Geometry: final body of the model. Coordinates: model frame, mm. Face numbers are marked on the shaded views. A direction names the side the tool comes from. Give positions to 0.01 mm unless a question says otherwise; leave off trailing zeros. Write each loop counter-clockwise with the first axis right and the second up, starting at its lowest first coordinate (ties: lowest second). Pieces come first, ordered by that corner, then holes. Notation, with made-up numbers: (27, 36) -> (65, 36) arc R15 cw to (65, 54) -> close; hole circle Ø7 at (16, 20). An arc over 180 degrees is marked (long way). Answer as a JSON object with one key per item and string values. Group by question number.
(1) Section query D-D on z = 5.25. Output: boundary loops of the cut face in (x, y), plus the area to 3 significant figures.
(2) Section query C-C on y = -4. Output: boundary loops of the cut face in (x, z), plus the area to 3 significant figures.
(3) Draft query along X for the marked faces 4, 5 and 6. Return one class per face: +X half, -X half, draft (parallel to the pull), parting line (faces both ways), or undercut.
(4) Material intervals for probe 1 along X at (y, z) = (-3, 3); probe 2 along Y at (x, z) = (5, 0.5); probe 3 along Z at (x, y) = (33.5, 5), sorted ascending.
(5) Contact query for flat-ended pins moving along their axis: pin 1 Ø5 at (x, z) = (22.5, 4) entering from +Y; pin 2 Ø1.9 at (x, y) = (32.5, 13.5) entering from -Z; pin 3 Ø3.5 at (x, y) = (12.5, 13.5) entering from +Z; pin 4 Ø17 at (x, y) = (13, 11.5) entering from +Z. Output: stop coordinate, or through.
(6) Section query B-B on y = 13.5. Output: boundary loops of the cut face in (x, z), plus the area to 3 significant figures.
(7) Section query A-A on x = 22.5. Output: boundary loops of the cut face in (y, z).
(8) Set-up query: the marked faces 1, 2 and 3. Return all of +Z, -Z, +X, -X, +Y, -Y with unobstructed straight access to the full face (end or side cutting, diameter ignored); none if empty.
from build123d import *

# Parameters (mm, degrees)
SALIENTE_EXTRUIR1_DEPTH = 45
REDONDEO1_R             = 2.5
CROQUIS2_R              = 2
CORTAR_EXTRUIR1_DEPTH   = 50.295030175
CROQUIS3_R              = 1.55
CORTAR_EXTRUIR2_DEPTH   = 53.242224302
CROQUIS4_W              = 45
CROQUIS4_H              = 18
SALIENTE_EXTRUIR2_DEPTH = 10
REDONDEO3_R             = 5
CROQUIS5_W              = 16
CROQUIS5_H              = 10
CORTAR_EXTRUIR3_DEPTH   = 53.242224302
REDONDEO4_R             = 5


with BuildPart() as part:
    # Croquis1 → Saliente-Extruir1 (new body)
    with BuildSketch(Plane(origin=(0, 0, 0), x_dir=(0, 0, -1), z_dir=(1, 0, 0))):
        Polygon((-9, -1.5), (9, -1.5), (9, 1.5), (9, 19.5), (6, 19.5), (6, 1.5), (-9, 1.5), align=None)
    extrude(amount=SALIENTE_EXTRUIR1_DEPTH)

    # Redondeo1
    redondeo1_edges = [part.edges().sort_by_distance(p)[0] for p in [
        (22.5, 1.5, -6),
    ]]
    fillet(redondeo1_edges, radius=REDONDEO1_R)

    # Croquis2 → Cortar-Extruir1 (cut, through all)
    with BuildSketch(Plane(origin=(0, 1.5, 0), x_dir=(1, 0, 0), z_dir=(0, 1, 0))):
        with Locations(Location((22.5, -4, 0), (0, 0, 270))):
            Circle(CROQUIS2_R)
    extrude(amount=-CORTAR_EXTRUIR1_DEPTH, mode=Mode.SUBTRACT)

    # Croquis3 → Cortar-Extruir2 (cut, through all)
    with BuildSketch(Plane(origin=(0, 0, -9), x_dir=(-1, 0, 0), z_dir=(0, 0, -1))):
        with Locations(Location((-32.5, 13.5, 0), (0, 0, 90))):
            Circle(CROQUIS3_R)
        with Locations((-12.5, 13.5)):
            Circle(CROQUIS3_R)
    extrude(amount=-CORTAR_EXTRUIR2_DEPTH, mode=Mode.SUBTRACT)

    # Croquis4 → Saliente-Extruir2 (add)
    with BuildSketch(Plane.XZ.offset(1.5)):
        with Locations((22.5, 0)):
            Rectangle(CROQUIS4_W, CROQUIS4_H)
    extrude(amount=SALIENTE_EXTRUIR2_DEPTH)

    # Redondeo3
    redondeo3_edges = [part.edges().sort_by_distance(p)[0] for p in [
        (45, -5, 9),
        (0, -5, 9),
    ]]
    fillet(redondeo3_edges, radius=REDONDEO3_R)

    # Croquis5 → Cortar-Extruir3 (cut, through all)
    with BuildSketch(Plane.XY.offset(9)):
        with Locations((22.5, -6.5)):
            Rectangle(CROQUIS5_W, CROQUIS5_H)
    extrude(amount=-CORTAR_EXTRUIR3_DEPTH, mode=Mode.SUBTRACT)

    # Redondeo4
    redondeo4_edges = [part.edges().sort_by_distance(p)[0] for p in [
        (45, 19.5, -7.5),
        (0, 19.5, -7.5),
    ]]
    fillet(redondeo4_edges, radius=REDONDEO4_R)


solid = part.part
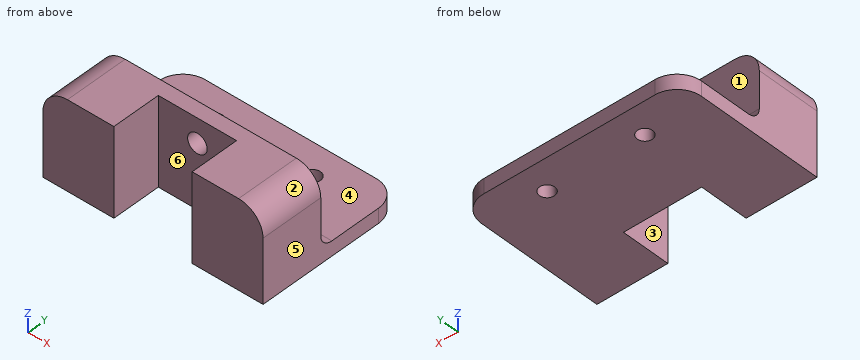
Answer list:
{
 "1": {"outline": "(0.16, -11.5) -> (14.5, -11.5) -> (14.5, -1.5) -> (20.94, -1.5) -> (20.94, 1.5) -> (0.16, 1.5) -> close; (24.06, -1.5) -> (30.5, -1.5) -> (30.5, -11.5) -> (44.84, -11.5) -> (44.84, 1.5) -> (24.06, 1.5) -> close", "area": "412 mm2"},
 "2": {"outline": "(0, -9) -> (14.5, -9) -> (14.5, 9) -> (5, 9) arc R5 ccw to (0, 4) -> close; (30.5, -9) -> (45, -9) -> (45, 4) arc R5 ccw to (40, 9) -> (30.5, 9) -> close", "area": "511 mm2"},
 "3": {"face 4": "draft", "face 5": "+X half", "face 6": "undercut"},
 "4": {"probe 1": "0 to 14.5, 30.5 to 45", "probe 2": "-11.5 to 1.5", "probe 3": "-9 to -6"},
 "5": {"pin 1": "y = 1.5", "pin 2": "through", "pin 3": "z = -6", "pin 4": "z = -5.79"},
 "6": {"outline": "(0, -9) -> (10.95, -9) -> (10.95, -6) -> (0, -6) -> close; (14.05, -9) -> (30.95, -9) -> (30.95, -6) -> (14.05, -6) -> close; (34.05, -9) -> (45, -9) -> (45, -6) -> (34.05, -6) -> close", "area": "116 mm2"},
 "7": {"outline": "(-1.5, -9) -> (19.5, -9) -> (19.5, -6) -> (4, -6) arc R2.5 cw to (1.5, -3.5) -> (1.5, 2) -> (-1.5, 2) -> close; (-1.5, 6) -> (1.5, 6) -> (1.5, 9) -> (-1.5, 9) -> close"},
 "8": {"face 1": "+Z, +X, -X, +Y", "face 2": "+Z, +X, +Y, -Y", "face 3": "+Z, -Z, -Y"}
}
